from build123d import *

# Parameters (mm, degrees)
SKETCH1_W           = 60
SKETCH1_H           = 30
BOSS_EXTRUDE2_DEPTH = 5
SKETCH2_R           = 11.5
BOSS_EXTRUDE3_DEPTH = 10
SKETCH3_R           = 8.69
CUT_EXTRUDE2_DEPTH  = 6
SKETCH4_R           = 1
CUT_EXTRUDE4_DEPTH  = 10


with BuildPart() as part:
    # Sketch1 → Boss-Extrude2 (new body)
    with BuildSketch(Plane.XY):
        Rectangle(SKETCH1_W, SKETCH1_H)
    extrude(amount=BOSS_EXTRUDE2_DEPTH)

    # Sketch2 → Boss-Extrude3 (add)
    with BuildSketch(Plane.XY.offset(5)):
        with Locations((-11.715, 0)):
            Circle(SKETCH2_R)
        with Locations((11.715, 0)):
            Circle(SKETCH2_R)
    extrude(amount=BOSS_EXTRUDE3_DEPTH)

    # Sketch3 → Cut-Extrude2 (cut)
    with BuildSketch(Plane.XY.offset(15)):
        with Locations((-11.715, 0)):
            Circle(SKETCH3_R)
        with Locations((11.715, 0)):
            Circle(SKETCH3_R)
    extrude(amount=-CUT_EXTRUDE2_DEPTH, mode=Mode.SUBTRACT)

    # Sketch4 → Cut-Extrude4 (cut)
    with BuildSketch(Plane.XY.offset(5)):
        with Locations((-25, 10)):
            Circle(SKETCH4_R)
        with Locations((25, 10)):
            Circle(SKETCH4_R)
        with Locations((25, -10)):
            Circle(SKETCH4_R)
        with Locations((-25, -10)):
            Circle(SKETCH4_R)
    extrude(amount=-CUT_EXTRUDE4_DEPTH, mode=Mode.SUBTRACT)


solid = part.part
CAD build for the part. Positions are in the model's coordinates, mm. A direction names the side the tool comes from. Round coordinates to 2 decimals unless told otherwise and drop trailing zeros. Order: outer loops, then holes, each group sorted by start corner. A loop starts at its lowest first (then second) coordinate and runs counter-clockwise, first axis right, second up. Notation, with made-up numbers: (41, -4) -> (100, -4) arc R11 ccw to (100, 15) -> close; hole circle Ø10 at (73, 30). An arc over 180 degrees is marked (long way). Write item = value, one per line. Start each with the question number.
(1) Which spindle directions (+Z, -Z, +X, -X, +Y, -Y) get a long thin tool onto all of the face, cutting with end or side? Do faces 1 (the flat face through (12, 0, 9)), 2 (the flat face through (0, 15, 2)). Say none if no direction does.
(2) Cut at C-C, the plane y = -10. List the corners of the cut face in (x, z), then the cut area to 3 significant figures.
(3) Cut at B-B, the plane z = 14.25. List the corners of the cut face in (x, y) (3 decimals), then the cut area to 3 significant figures.
(4) Pull direction Y, two halves, no side cores. Call faces 3 (the flat face through (0, -15, 2)), 4 (the cylindrical face through (-25, -9, 3)), 5 (the cylindrical face through (-25, 11, 3)), 6 (the flat face through (-10, 9, 15)): released by +Y, released by -Y, zero draft, split by the parting line, or undercut.
(5) Probe line 1 (Y direction, x = 25, z = 1.85); line 2 (Z direction, x = -26.5, y = 3); line 3 (Z direction, x = -17, y = 3.5). List the from-to ranges inside material, lowest first. Write a range as [from, to].
(6) Cut at D-D, the plane x = -13. List the corners of the cut face in (y, z).
(7) Pin check, flat tips, straight feed: P1, Ø5, axis at x = 13.5, y = 1, coming from the +Z side; P2, Ø1.5, axis at x = 9, z = 6, coming from the +Y side; P3, Ø3, axis at x = -25, y = -10, coming from the +Z side; P4, Ø1.6, axis at x = 25, y = 10, coming from the +Z side. Stop position of each tip, or through.
(8) Cut at A-A, the plane x = 25. List the corners of the cut face in (y, z).
Model answer:
q1.face_1 = +Z
q1.face_2 = +Z, -Z, +X, -X, +Y
q2.outline = (-30, 0) -> (-26, 0) -> (-26, 5) -> (-30, 5) -> close; (-24, 0) -> (24, 0) -> (24, 5) -> (17.39, 5) -> (17.39, 15) -> (6.04, 15) -> (6.04, 5) -> (-6.04, 5) -> (-6.04, 15) -> (-17.39, 15) -> (-17.39, 5) -> (-24, 5) -> close; (26, 0) -> (30, 0) -> (30, 5) -> (26, 5) -> close
q2.area = 507 mm2
q3.outline = circle Ø23 at (-11.715, 0); circle Ø23 at (11.715, 0); hole circle Ø17.38 at (-11.715, 0); hole circle Ø17.38 at (11.715, 0)
q3.area = 356 mm2
q4.face_3 = released by -Y
q4.face_4 = undercut
q4.face_5 = undercut
q4.face_6 = zero draft
q5.line_1 = [-15, -11], [-9, 9], [11, 15]
q5.line_2 = [0, 5]
q5.line_3 = [0, 9]
q6.outline = (-15, 0) -> (15, 0) -> (15, 5) -> (11.43, 5) -> (11.43, 15) -> (8.59, 15) -> (8.59, 9) -> (-8.59, 9) -> (-8.59, 15) -> (-11.43, 15) -> (-11.43, 5) -> (-15, 5) -> close
q7.P1 = 9
q7.P2 = 11.33
q7.P3 = 5
q7.P4 = through
q8.outline = (-15, 0) -> (-11, 0) -> (-11, 5) -> (-15, 5) -> close; (-9, 0) -> (9, 0) -> (9, 5) -> (-9, 5) -> close; (11, 0) -> (15, 0) -> (15, 5) -> (11, 5) -> close
